```python
from build123d import *

# Parameters (mm, degrees)
F1_DEPTH = 30
F2_R     = 7.5
F3_DEPTH = 66.5296831478
F4_SIZE  = 5


with BuildPart() as f1:
    # F0 (on Top) → F1 (new body)
    with BuildSketch(Plane.XY):
        with BuildLine():
            Line((-6.9337203167, 2.2713398635), (-46.9337203167, 2.2713398635))
            Line((-46.9337203167, 2.2713398635), (-46.9337203167, -39.7286601365))
            Line((-46.9337203167, -39.7286601365), (-6.9337203167, -39.7286601365))
            Line((-6.9337203167, -39.7286601365), (-6.9337203167, -17.885550487))
            Line((-6.9337203167, -17.885550487), (16.2017301439, -4.3453868678))
            ThreePointArc((16.2017301439, -4.3453868678), (58.3330589287, 22.2213546523), (12.2138993907, 3.4100882496))
            Line((12.2138993907, 3.4100882496), (-6.9337203167, -6.4725532874))
            Line((-6.9337203167, -6.4725532874), (-6.9337203167, 2.2713398635))
        make_face()
    extrude(amount=F1_DEPTH)

    # F2 (on face) → F3 (cut, through all)
    with BuildSketch(Plane(origin=(6.027939026, -10.2996602284, 0), x_dir=(0.8630557619, 0.5051086534, 0), z_dir=(0.5051086534, -0.8630557619, 0))):
        with Locations((-2.7203583159, 17.3664018512)):
            Circle(F2_R)
    extrude(amount=-F3_DEPTH, mode=Mode.SUBTRACT)

    # F4
    f4_edges = [f1.edges().sort_by_distance(p)[0] for p in [
        (58.333059, 22.221355, 30),
        (-26.93372, 2.27134, 30),
    ]]
    chamfer(f4_edges, length=F4_SIZE)


solid = f1.part
```
The model under review builds one solid part; all positions refer to its coordinate system, in mm. A direction names the side the tool comes from. Give positions to 0.01 mm unless a question says otherwise; leave off trailing zeros. Write each loop counter-clockwise with the first axis right and the second up, starting at its lowest first coordinate (ties: lowest second). Pieces come first, ordered by that corner, then holes. Notation, with made-up numbers: (-8.5, -40) - (1.5, -40) arc R28 ccw to (1.5, -21) - close; hole circle Ø1 at (86.5, 89.5). An arc over 180 degrees is marked (long way). Answer in a Markdown table with one row per item. Add a question column.
1. We need section A-A on z = 12.5. Write out the cut boundary in (x, y).
2. We need section C-C on z = 7. Write out the cut boundary in (x, y), then the cut area to 3 significant figures.
3. We need section D-D on z = 19.5. Write out the cut boundary in (x, y).
4. Tool access review of faces 1 (the cylindrical face through (58.79, 21.29, 12.32)), 2 (the flat face through (-26.654, -0.264, 27.535)), 3 (the flat face through (-27, 2.271, 12)): name each direction out of +Z, -Z, +X, -X, +Y, -Y from which nothing blocks a thin tool from reaching the whole face with its end or side.
5. We need section B-B on x = -21. Write out the cut boundary in (y, z).
6. Draft analysis for pull direction X (two halves, no side actions). For faces 4 (the cylindrical face through (-6.75, -8.686, 17.696)), 5 (the flat face through (-6.934, -29, 15)), 6 (the flat face through (6, -1, 0)), state which applies: +X half, -X half, draft (parallel to the pull), parting line (faces both ways), or undercut.
7. Insertion check: P1, Ø10, axis at x = -6, y = -24, coming from the -Z side; P2, Ø4.5, axis at y = -1, z = 27.5, coming from the +X side; P3, Ø5, axis at y = 7.5, z = 23, coming from the +X side; P4, Ø7.5, axis at x = -21, z = 14.5, coming from the +Y side. Each pin has a flat end and moves straight along its axis. Give the tip position at first contact, or say it passes through.
8. Wall thickness on line 1 along Y through (x, z) = (-35.5, 9.5); line 2 along Y through (x, z) = (36.5, 5.5); line 3 along X through (y, z) = (-20, 8): over which ranges is each line inside the solid? List them lowest first. Write a range as [from, to].
Ans:
| question | item | result |
|---|---|---|
| 1 | outline | (-46.93, -39.73) - (-6.93, -39.73) - (-6.93, -17.89) - (-1.25, -14.56) - (-6.2, -6.09) - (-6.93, -6.47) - (-6.93, -4.84) - (-11.09, 2.27) - (-46.93, 2.27) - close; (3.96, -0.85) - (8.61, -8.79) - (16.2, -4.35) arc R25 ccw (long way) to (12.21, 3.41) - close |
| 2 | outline | (-46.93, -39.73) - (-6.93, -39.73) - (-6.93, -17.89) - (16.2, -4.35) arc R25 ccw (long way) to (12.21, 3.41) - (-6.93, -6.47) - (-6.93, 2.27) - (-46.93, 2.27) - close |
| 2 | area | 3,870 mm^2 |
| 3 | outline | (-46.93, -39.73) - (-6.93, -39.73) - (-6.93, -17.89) - (-2.53, -15.31) - (-12.81, 2.27) - (-46.93, 2.27) - close; (5.28, -0.17) - (9.89, -8.04) - (16.2, -4.35) arc R25 ccw (long way) to (12.21, 3.41) - close |
| 4 | face 1 | +Z, -Z |
| 4 | face 2 | +Z, -X, +Y |
| 4 | face 3 | +Z, -Z, -X, +Y |
| 5 | outline | (-39.73, 0) - (2.27, 0) - (2.27, 25) - (-2.73, 30) - (-39.73, 30) - close |
| 6 | face 4 | undercut |
| 6 | face 5 | +X half |
| 6 | face 6 | draft |
| 7 | P1 | stops at z = 0 |
| 7 | P2 | stops at x = 58.12 |
| 7 | P3 | stops at x = 61.09 |
| 7 | P4 | stops at y = 2.27 |
| 8 | line 1 | y = [-39.73, 2.27] |
| 8 | line 2 | y = [-14.21, 35.79] |
| 8 | line 3 | x = [-46.93, -6.93] |
